Read the model definition and answer for the solid it produces. Units are mm, in the model's axes. A direction names the side the tool comes from. Give positions to 0.01 mm unless a question says otherwise; leave off trailing zeros. Order: outer loops, then holes, each group sorted by start corner. A loop starts at its lowest first (then second) coordinate and runs counter-clockwise, first axis right, second up. Notation, with made-up numbers: (54.25, 70.25) - (75.25, 70.25) arc R19 cw to (75.25, 102.25) - close; hole circle Ø6 at (69.5, 79.25). An arc over 180 degrees is marked (long way). Use a Markdown table: item, result. Add a question column.
1. A cutting plane is placed at D-D on z = 35.5. Determine the outline of the cut face in (x, y).
2. A cutting plane is placed at C-C on y = 1.5. State how many separate pieces and enclosed holes the cut face has, and give its area (3 significant figures).
3. A cutting plane is placed at B-B on x = -35. Determine the outline of the cut face in (y, z).
4. Which of the six approach directions +Z, -Z, +X, -X, +Y, -Y give full straight-line access (tool end or side, diameter ignored) to faces 5 (the flat face through (-1, 0, 0)), 6 (the cylindrical face through (-2.343, 17.847, 34.79))?
5. Consider L1, parallel to Y at x = 0, z = 45; L2, parallel to Z at x = 17, y = 12; L3, parallel to Y at x = 30.5, z = 5. Determine where each line is inside the solid, lowest interval first.
6. Flat-ended cylindrical pins translate along their axes: P1, Ø8, axis at x = -33.5, z = 15, coming from the -Y side; P2, Ø6, axis at x = 29, z = 25.5, coming from the -Y side; P3, Ø3, axis at x = 27.5, y = -1, coming from the +Z side; P4, Ø10.5, axis at x = 0, y = 0, coming from the +Z side. Find the tip coordinate at first contact, or state that the pin passes through.
7. For a pull along Y with two mould halves and no side action, classify faces 1 (the cylindrical face through (-30, 0, 10)), 2 (the flat face through (-25.2, -15.717, 9.86)), 3 (the conical face through (-0.329, -1.483, 20.656)), 4 (the flat face through (-4, -8, 50)) as released by +Y, released by -Y, zero draft, split by the parting line, or undercut.
8. A cutting plane is placed at A-A on z = 7.5. Determine the outline of the cut face in (x, y).
```python
from build123d import *

# Parameters (mm, degrees)
F1_DEPTH = 20
F3_D     = 10
F3_DEPTH = 20
F3_TIP   = 3.0043030951
F4_R     = 18
F5_DEPTH = 30
F7_D     = 17.5
F7_DEPTH = 25
F7_TIP   = 5.2575304165


with BuildPart() as f1:
    # F0 (on Top) → F1 (new body)
    with BuildSketch(Plane.XY):
        with BuildLine():
            Line((10.714285677, -22.587697541), (39.2857142338, -9.0350790325))
            ThreePointArc((39.2857142338, -9.0350790325), (44.9999999554, 0), (39.2857142338, 9.0350790325))
            Line((39.2857142338, 9.0350790325), (10.714285677, 22.587697541))
            ThreePointArc((10.714285677, 22.587697541), (2.52e-08, 24.9999999554), (-10.7142856314, 22.5876975626))
            Line((-10.7142856314, 22.5876975626), (-39.2857142793, 9.0350790815))
            ThreePointArc((-39.2857142793, 9.0350790815), (-45.0000000446, 0), (-39.2857142793, -9.0350790815))
            Line((-39.2857142793, -9.0350790815), (-10.7142856314, -22.5876975626))
            ThreePointArc((-10.7142856314, -22.5876975626), (2.52e-08, -24.9999999554), (10.714285677, -22.587697541))
        make_face()
    extrude(amount=F1_DEPTH)

    # F3
    with Locations(Plane.XY.offset(20)):
        with Locations((-35, 0), (35, 0)):
            Hole(F3_D / 2, depth=F3_DEPTH)
            with Locations((0, 0, -(F3_DEPTH + F3_TIP / 2))):  # 118° drill point
                Cone(0, F3_D / 2, F3_TIP, mode=Mode.SUBTRACT)

    # F4 (on face) → F5 (join)
    with BuildSketch(Plane.XY.offset(20)):
        Circle(F4_R)
    extrude(amount=F5_DEPTH)

    # F7
    with Locations(Plane.XY.offset(50)):
        with Locations((0, 0)):
            Hole(F7_D / 2, depth=F7_DEPTH)
            with Locations((0, 0, -(F7_DEPTH + F7_TIP / 2))):  # 118° drill point
                Cone(0, F7_D / 2, F7_TIP, mode=Mode.SUBTRACT)


solid = f1.part
```
Output values:
| question | item | result |
|---|---|---|
| 1 | outline | circle Ø36 at (0, 0); hole circle Ø17.5 at (0, 0) |
| 2 | separate pieces | 3 |
| 2 | enclosed holes | 0 |
| 2 | area | 2,020 mm² |
| 3 | outline | (-11.07, 0) - (-5, 0) - (-5, 20) - (-11.07, 20) - close; (5, 0) - (11.07, 0) - (11.07, 20) - (5, 20) - close |
| 4 | face 5 | -Z, +X, -X, +Y, -Y |
| 4 | face 6 | +Z |
| 5 | L1 | -18 to -8.75, 8.75 to 18 |
| 5 | L2 | 0 to 20 |
| 5 | L3 | -13.2 to -2.18, 2.18 to 13.2 |
| 6 | P1 | y = -13.68 |
| 6 | P2 | through |
| 6 | P3 | z = 20 |
| 6 | P4 | z = 22.9 |
| 7 | face 1 | undercut |
| 7 | face 2 | released by -Y |
| 7 | face 3 | undercut |
| 7 | face 4 | zero draft |
| 8 | outline | (-39.29, -9.04) - (-10.71, -22.59) arc R25 ccw to (10.71, -22.59) - (39.29, -9.04) arc R10 ccw to (39.29, 9.04) - (10.71, 22.59) arc R25 ccw to (-10.71, 22.59) - (-39.29, 9.04) arc R10 ccw to start; hole circle Ø10 at (-35, 0); hole circle Ø10 at (35, 0) |
